Source: CAD feature listing. Evaluate the final solid. Frame: model axes, mm. Face numbers are marked on the shaded views. Coordinates: 2 decimals unless noted, no trailing zeros. Order: outer loops, then holes, each group sorted by start corner. A loop starts at its lowest first (then second) coordinate and runs counter-clockwise, first axis right, second up. Notation, with made-up numbers: (27.5, 30.25) -> (31.5, 30.25) arc R15 ccw to (31.5, 46.25) -> close; hole circle Ø2 at (-11, 15). An arc over 180 degrees is marked (long way). Put each result on its own line as item: value.
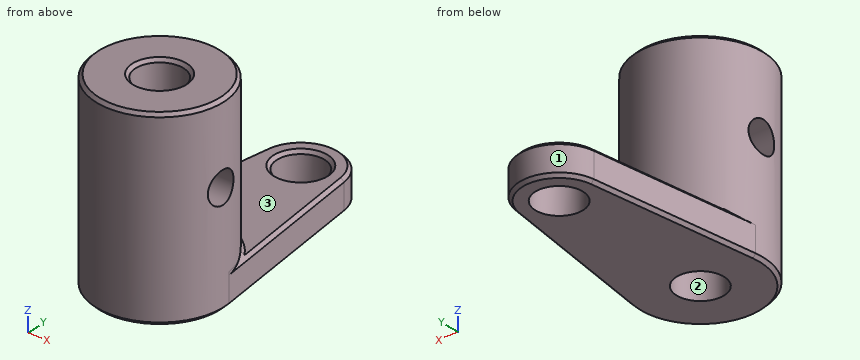
from build123d import *

# Parameters (mm, degrees)
SKETCH1_R               = 1.5
BOSS_EXTRUDE1_DEPTH     = 2
SKETCH2_R               = 4
SKETCH2_R_2             = 1.5
BOSS_EXTRUDE2_DEPTH     = 10
CUT_EXTRUDE1_DEPTH      = 19.5
CUT_EXTRUDE1_DEPTH_BACK = 19.5
SKETCH3_R               = 1
CHAMFER1_SIZE           = 0.2
CHAMFER2_SIZE           = 0.2


with BuildPart() as part:
    # Sketch1 → Boss-Extrude1 (new body)
    with BuildSketch(Plane.XY):
        with BuildLine():
            Line((-2.476647127, 11.340909091), (-3.962635403, 0.545454545))
            ThreePointArc((-3.962635403, 0.545454545), (0, -4), (3.962635403, 0.545454545))
            Line((3.962635403, 0.545454545), (2.476647127, 11.340909091))
            ThreePointArc((2.476647127, 11.340909091), (0, 13.5), (-2.476647127, 11.340909091))
        make_face()
        with Locations((0, 11)):
            Circle(SKETCH1_R, mode=Mode.SUBTRACT)
        Circle(SKETCH1_R, mode=Mode.SUBTRACT)
    extrude(amount=BOSS_EXTRUDE1_DEPTH)

    # Sketch2 → Boss-Extrude2 (add)
    with BuildSketch(Plane.XY.offset(2)):
        with Locations(Location((0, 0, 0), (0, 0, 172.162520237))):
            Circle(SKETCH2_R)
        Circle(SKETCH2_R_2, mode=Mode.SUBTRACT)
    extrude(amount=BOSS_EXTRUDE2_DEPTH)

    # Sketch3 → Cut-Extrude1 (cut, two sides: drawn at the far end of the back side and taken through both)
    with BuildSketch(Plane(origin=(0, 0, 0), x_dir=(0, 0, -1), z_dir=(1, 0, 0)).offset(-CUT_EXTRUDE1_DEPTH_BACK)):
        with Locations((-7, 0)):
            Circle(SKETCH3_R)
    extrude(amount=CUT_EXTRUDE1_DEPTH + CUT_EXTRUDE1_DEPTH_BACK, mode=Mode.SUBTRACT)

    # Chamfer1
    # the kernel refuses this chamfer: 0.2 mm, written as the material it takes off along each edge
    with BuildSketch(Plane(origin=(0, 11, 2), x_dir=(1, 0, 0), z_dir=(0, -1, 0))) as chamfer1_piece_1:
        Polygon((1.5 + CHAMFER1_SIZE, 0), (1.5, -CHAMFER1_SIZE), (1.5, 0), align=None)
    revolve(axis=Axis((0, 11, 2), (0, 0, 1)), mode=Mode.SUBTRACT)
    with BuildSketch(Plane(origin=(0, 11, 2), x_dir=(0.9906588508046985, 0.13636363636363596, 0), z_dir=(0.13636363636363596, -0.9906588508046985, 0))) as chamfer1_piece_2:
        Polygon((2.5, -CHAMFER1_SIZE), (2.5 - CHAMFER1_SIZE, 0), (2.5, 0), align=None)
    revolve(axis=Axis((0, 11, 2), (0, 0, 1)), revolution_arc=164.325040474, mode=Mode.SUBTRACT)
    with BuildSketch(Plane(origin=(-2.476647127, 11.340909091, 2), x_dir=(0.9902842994465351, -0.13631207957881322, 0.02749587661058738), z_dir=(-0.1363636363636364, -0.9906588508046986, 0))) as chamfer1_piece_3_section:
        Polygon((CHAMFER1_SIZE * 0.999621916911, -CHAMFER1_SIZE * 0.0274958766106), (-CHAMFER1_SIZE * 0.0274958766106, -CHAMFER1_SIZE * 0.999621916911), (0, 0), align=None)
    chamfer1_piece_3 = extrude(amount=11.411583956, mode=Mode.PRIVATE)
    chamfer1_piece_3 = chamfer1_piece_3 - Plane(origin=(0, 0, 1.932985059), x_dir=(-0.9906588508048991, 0.13636363636217924, 0), z_dir=(0, 0, -1)) * Cylinder(4, 24, mode=Mode.PRIVATE)
    add(chamfer1_piece_3, mode=Mode.SUBTRACT)
    with BuildSketch(Plane(origin=(0, 0, 12), x_dir=(-0.9906588508048991, 0.13636363636217924, 0), z_dir=(0.13636363636217924, 0.9906588508048991, 0))) as chamfer1_piece_4:
        Polygon((4, -CHAMFER1_SIZE), (4 - CHAMFER1_SIZE, 0), (4, 0), align=None)
    revolve(axis=Axis((0, 0, 12), (0, 0, 1)), mode=Mode.SUBTRACT)
    with BuildSketch(Plane(origin=(0, 0, 12), x_dir=(1, 0, 0), z_dir=(0, -1, 0))) as chamfer1_piece_5:
        Polygon((1.5, -CHAMFER1_SIZE), (1.5 + CHAMFER1_SIZE, 0), (1.5, 0), align=None)
    revolve(axis=Axis((0, 0, 12), (0, 0, 1)), mode=Mode.SUBTRACT)
    with BuildSketch(Plane(origin=(-2.476647127, 11.340909091, 0), x_dir=(0.9902842994465351, -0.13631207957881322, -0.027495876610586414), z_dir=(-0.1363636363636364, -0.9906588508046986, 0))) as chamfer1_piece_6:
        Polygon((CHAMFER1_SIZE * 0.999621916911, CHAMFER1_SIZE * 0.0274958766106), (-CHAMFER1_SIZE * 0.0274958766106, CHAMFER1_SIZE * 0.999621916911), (0, 0), align=None)
    extrude(amount=10.897247359, mode=Mode.SUBTRACT)
    with BuildSketch(Plane(origin=(0, 11, 0), x_dir=(0.9906588508046985, 0.13636363636363596, 0), z_dir=(0.13636363636363596, -0.9906588508046985, 0))) as chamfer1_piece_7:
        Polygon((2.5, CHAMFER1_SIZE), (2.5 - CHAMFER1_SIZE, 0), (2.5, 0), align=None)
    revolve(axis=Axis((0, 11, 0), (0, 0, 1)), revolution_arc=164.325040474, mode=Mode.SUBTRACT)
    with BuildSketch(Plane(origin=(3.962635403, 0.545454545, 0), x_dir=(0.027239033524910743, 0.0037494377196253415, 0.9996219169112968), z_dir=(-0.1363636363636364, 0.9906588508046986, 0))) as chamfer1_piece_8:
        Polygon((CHAMFER1_SIZE * 0.999621916911, -CHAMFER1_SIZE * 0.0274958766106), (-CHAMFER1_SIZE * 0.0274958766106, -CHAMFER1_SIZE * 0.999621916911), (0, 0), align=None)
    extrude(amount=10.897247359, mode=Mode.SUBTRACT)
    with BuildSketch(Plane(origin=(0, 0, 0), x_dir=(-0.9906588508046986, 0.13636363636363646, 0), z_dir=(0.13636363636363646, 0.9906588508046986, 0))) as chamfer1_piece_9:
        Polygon((4, CHAMFER1_SIZE), (4 - CHAMFER1_SIZE, 0), (4, 0), align=None)
    revolve(axis=Axis((0, 0, 0), (0, 0, 1)), revolution_arc=195.674959526, mode=Mode.SUBTRACT)
    with BuildSketch(Plane(origin=(4.032772212, 0.035922443, 2), x_dir=(0.02723903352491077, 0.003749437719625345, -0.9996219169112968), z_dir=(-0.1363636363636364, 0.9906588508046986, 0))) as chamfer1_piece_10_section:
        Polygon((CHAMFER1_SIZE * 0.999621916911, CHAMFER1_SIZE * 0.0274958766106), (-CHAMFER1_SIZE * 0.0274958766106, CHAMFER1_SIZE * 0.999621916911), (0, 0), align=None)
    chamfer1_piece_10 = extrude(amount=11.411583956, mode=Mode.PRIVATE)
    chamfer1_piece_10 = chamfer1_piece_10 - Plane(origin=(0, 0, 1.932985114), x_dir=(-0.9906588508048991, 0.13636363636217924, 0), z_dir=(0, 0, -1)) * Cylinder(4, 24, mode=Mode.PRIVATE)
    add(chamfer1_piece_10, mode=Mode.SUBTRACT)

    # Chamfer2
    # the kernel refuses this chamfer: 0.2 mm, written as the material it adds along each edge
    with BuildSketch(Plane(origin=(0, 0, 2), x_dir=(0.9474392315450817, 0.31993577875765195, 0), z_dir=(0.31993577875765195, -0.9474392315450817, 0))) as chamfer2_piece_1_section:
        Polygon((4 + CHAMFER2_SIZE, 0), (4, CHAMFER2_SIZE), (4, 0), align=None)
    chamfer2_piece_1 = revolve(axis=Axis((0, 0, 2), (0, 0, 1)), revolution_arc=142.681917796, mode=Mode.PRIVATE)
    chamfer2_piece_1 = split(chamfer2_piece_1, bisect_by=Plane(origin=(1.558048565, 4.310442532, 3.668717781), z_dir=(-0.700501591246356, -0.0964236519801952, -0.7071067811866362)), keep=Keep.TOP, mode=Mode.PRIVATE)
    chamfer2_piece_1 = split(chamfer2_piece_1, bisect_by=Plane(origin=(-1.558048565, 4.310442532, 3.668717781), z_dir=(0.7005015912467089, -0.09642365198024379, -0.70710678118628)), keep=Keep.TOP, mode=Mode.PRIVATE)
    add(chamfer2_piece_1)


solid = part.part
1. Cut plane A-A on y = 0. Output: boundary loops of the cut face in (x, z), plus the area to 3 significant figures.
Numbers:
outline: (-4, 0.2) -> (-3.8, 0) -> (-1.5, 0) -> (-1.5, 6) -> (-4, 6) -> close; (-4, 8) -> (-1.5, 8) -> (-1.5, 11.8) -> (-1.7, 12) -> (-3.8, 12) -> (-4, 11.8) -> close; (1.5, 0) -> (3.8, 0) -> (4, 0.2) -> (4, 6) -> (1.5, 6) -> close; (1.5, 8) -> (4, 8) -> (4, 11.8) -> (3.8, 12) -> (1.7, 12) -> (1.5, 11.8) -> close
area: 49.9 mm2
2. Ray query, line 1 along Y through (x, z) = (0, 7.5); line 2 along Z through (x, y) = (-1.5, 12.75). Return the intervals inside material, ascending.
Numbers:
line 1: y = -4 to -1.5, 1.5 to 4
line 2: z = 0 to 2
3. Pull-direction query (Y, two-part tool) for the marked faces 1, 2 and 3; classes: pulls with the +Y half, pulls with the -Y half, needs draft (parallel to the pull), parting line crosses it, or undercut.
Numbers:
face 1: pulls with the +Y half
face 2: undercut
face 3: needs draft
4. Cut plane C-C on z = 7. Output: boundary loops of the cut face in (x, y).
Numbers:
outline: (-3.87, -1) arc R4 ccw to (3.87, -1) -> (1.12, -1) arc R1.5 cw to (-1.12, -1) -> close; (-3.87, 1) -> (-1.12, 1) arc R1.5 cw to (1.12, 1) -> (3.87, 1) arc R4 ccw to start
5. First-contact query: pin 1 (3 mm diameter, centred on x = 2.5, z = 9.5, fed in from +Y); pin 2 (2 mm diameter, centred on y = 2.5, z = 9.5, fed in from -X); pin 3 (2 mm diameter, centred on x = -0.5, y = 8, fed in from +Z); pin 4 (2 mm diameter, centred on y = 6.5, z = 6, fed in from -X). Flat tips, straight axial feed; report the tip coordinate or a pass-through.
Numbers:
pin 1: stops at y = 3.87
pin 2: stops at x = -3.71
pin 3: stops at z = 2
pin 4: passes through
6. Cut plane B-B on x = 0. Output: boundary loops of the cut face in (y, z).
Numbers:
outline: (-4, 0.2) -> (-3.8, 0) -> (-1.5, 0) -> (-1.5, 11.8) -> (-1.7, 12) -> (-3.8, 12) -> (-4, 11.8) -> close; (1.5, 0) -> (9.5, 0) -> (9.5, 1.8) -> (9.3, 2) -> (4.2, 2) -> (4, 2.2) -> (4, 11.8) -> (3.8, 12) -> (1.7, 12) -> (1.5, 11.8) -> close; (12.5, 0) -> (13.3, 0) -> (13.5, 0.2) -> (13.5, 1.8) -> (13.3, 2) -> (12.7, 2) -> (12.5, 1.8) -> close
7. Cut plane D-D on y = 11. Output: boundary loops of the cut face in (x, z), plus the area to 3 significant figures.
Numbers:
outline: (-2.52, 0.2) -> (-2.32, 0) -> (-1.5, 0) -> (-1.5, 1.8) -> (-1.7, 2) -> (-2.32, 2) -> (-2.52, 1.8) -> close; (1.5, 0) -> (2.32, 0) -> (2.52, 0.2) -> (2.52, 1.8) -> (2.32, 2) -> (1.7, 2) -> (1.5, 1.8) -> close
area: 3.97 mm2
